Part model, mm, in its own coordinate system. A direction names the side the tool comes from. Coordinates: 2 decimals unless noted, no trailing zeros. Loops run counter-clockwise (first coordinate to the right, second up) from the corner with the lowest first, then second, coordinate; pieces in that order, holes last. Notation, with made-up numbers: (53.5, 89.25) -> (72.5, 89.25) arc R26 ccw to (72.5, 106.25) -> close; hole circle Ø7 at (49, 14.5). An arc over 180 degrees is marked (long way). Use one line per item in the form item = value. Start each with the question number.
(1) Drill centre lines: L1, parallel to Y at x = 3.75, z = -0.55; L2, parallel to X at y = 0.6, z = 2.05; L3, parallel to X at y = 2.3, z = 1.8. Where is each one in solid material? Low to high. Write a range as [from, to].
(2) Pin check, flat tips, straight feed: P1, Ø1.5, axis at x = -0.5, y = 2, coming from the -Z side; P2, Ø1.5, axis at y = -0.5, z = 1.5, coming from the +X side. Stop position of each tip, or through.
(3) Mould opens along Z. For faces 1 (the flat face through (8.3, 0, 0)), 2 (the cylindrical face through (4.21, -1.5, 0.07)), 3 (the flat face through (-1.28, -0.87, 0.49)), 4 (the flat face through (-1.28, 0.87, -0.49)) say: +Z half, -Z half, draft (parallel to the pull), parting line (faces both ways), or undercut.
(4) Band-saw the part on A-A on x = 6.25. Give the cut face in (y, z), then the cut area to 3 significant figures.
(5) 3-axis set-ups, long thin cutter, end or side, ignore diameter. For faces 5 (the flat face through (-1.7, 0, -1.3)), 6 (the flat face through (-1.28, -0.86, -0.51)): which of +Z, -Z, +X, -X, +Y, -Y reach the whole face in a straight line?
```python
from build123d import *

# Parameters (mm, degrees)
CUT_EXTRUDE1_DEPTH = 0.85


with BuildPart() as part:
    # Sketch1 → Revolve1 (revolve)
    with BuildSketch(Plane.XY):
        Polygon((-1.7, 0), (-1.7, 3), (-1.5, 3), (0, 1.5), (8.3, 1.5), (8.3, 0), align=None)
    revolve(axis=Axis((-1.7, 0, 0), (1, 0, 0)))

    # Sketch2 → Cut-Revolve2 (revolve, cut)
    with BuildSketch(Plane.XY):
        Polygon((-0.249139381, 0), (-0.85, 1), (-1.7, 1), (-1.7, 0), align=None)
    revolve(axis=Axis((-0.249139381, 0, 0), (-1, 0, 0)), mode=Mode.SUBTRACT)

    # Sketch3 → Cut-Extrude1 (cut)
    with BuildSketch(Plane.ZY.offset(1.7)):
        Polygon((0, 1.154700538), (-1, 0.577350269), (-1, -0.577350269), (0, -1.154700538), (1, -0.577350269), (1, 0.577350269), align=None)
    extrude(amount=-CUT_EXTRUDE1_DEPTH, mode=Mode.SUBTRACT)


solid = part.part
```
A:
q1.L1 = [-1.4, 1.4]
q1.L2 = [-1.7, -0.64]
q1.L3 = [-1.7, -1.42]
q2.P1 = -2.09
q2.P2 = 8.3
q3.face_1 = draft
q3.face_2 = parting line
q3.face_3 = undercut
q3.face_4 = undercut
q4.outline = circle Ø3 at (0, 0)
q4.area = 7.07 mm²
q5.face_5 = +Z, -Z, -X, +Y, -Y
q5.face_6 = -X
